Input: part model. Units: mm. Frame: model coordinates. Round coordinates to 2 decimals unless told otherwise and drop trailing zeros. Write each loop counter-clockwise with the first axis right and the second up, starting at its lowest first coordinate (ties: lowest second). Pieces come first, ordered by that corner, then holes. Notation, with made-up numbers: (83.25, -35) -> (136.25, -35) arc R15 cw to (136.25, -28) -> close; hole circle Ø11 at (31.25, 87). An arc over 180 degrees is marked (long way). Write item = value, one per line.
```python
from build123d import *

# Parameters (mm, degrees)
EXTRUDE_1_DEPTH = 10


with BuildPart() as part:
    # Эскиз1_fr → Бобышка-Вытянуть1 (new body)
    with BuildSketch(Plane.XY):
        with BuildLine():
            Line((0, 0), (0, 20))
            add(Edge.make_bspline(
                [(0, 20), (0, 38.146025899), (-14.209474182, 48.611098897), (-41.986949672, 54.649680525)],
                knots=[0, 0, 0, 0, 1, 1, 1, 1], degree=3))
            Line((-41.986949672, 54.649680525), (-103.301225383, 67.978870897))
            add(Edge.make_bspline(
                [(-103.301225383, 67.978870897), (-115.500001367, 70.63077872), (-131.292525164, 63.393306184), (-131.292525164, 43.097715536)],
                knots=[0, 0, 0, 0, 1, 1, 1, 1], degree=3))
            Line((-131.292525164, 43.097715536), (-131.292525164, 0))
            add(Edge.make_bspline(
                [(-97.969549234, -25.769768053), (-112.011160689, -25.769768053), (-131.292525164, -19.025155818), (-131.292525164, 0)],
                knots=[0, 0, 0, 0, 1, 1, 1, 1], degree=3))
            Line((-97.969549234, -25.769768053), (-33.545129103, -25.769768053))
            add(Edge.make_bspline(
                [(-33.545129103, -25.769768053), (-19.444866568, -25.769768053), (0, -19.063757455), (0, 0)],
                knots=[0, 0, 0, 0, 1, 1, 1, 1], degree=3))
        make_face()
    extrude(amount=EXTRUDE_1_DEPTH)


solid = part.part
```
1) Cut plane A-A (x = -75). Return the cut outline in (y, z), and give its area (3 significant figures).
Solutions:
outline = (-25.77, 0) -> (61.83, 0) -> (61.83, 10) -> (-25.77, 10) -> close
area = 876 mm^2
2) First-contact query: P1, Ø1, axis at y = -6, z = 8.5, coming from the +X side. Flat tip, straight axial feed; report the tip coordinate or a pass-through.
Solutions:
P1 = -0.59
3) Cut plane B-B (x = -89). Return the cut outline in (y, z).
Solutions:
outline = (-25.77, 0) -> (64.87, 0) -> (64.87, 10) -> (-25.77, 10) -> close
4) Line query: L1, parallel to Y at x = -107, z = 5; L2, parallel to Y at x = -80.5, z = 7.5; L3, parallel to X at y = -3.5, z = 7.25. Output: solid intervals per line, ascending. Write a range as from..to.
Solutions:
L1 = -24.88..68.47
L2 = -25.77..63.02
L3 = -131.06..-0.23
